Geometry check sheet. Reference: the model listing, model coordinates, mm. Round coordinates to 2 decimals unless told otherwise and drop trailing zeros. Write each loop counter-clockwise with the first axis right and the second up, starting at its lowest first coordinate (ties: lowest second). Pieces come first, ordered by that corner, then holes. Notation, with made-up numbers: M 74,89 L 96,89 A22 ccw 96,110 Z; hole C 28,37 d7. An arc over 180 degrees is marked long. Use a Markdown table: item, result.
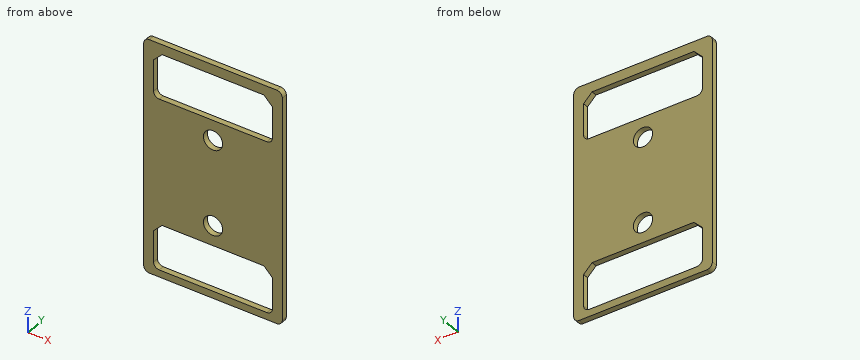
Autodesk Inventor part; units mm, degrees
ref_plane "YZ Plane" through (0, 0, 0) normal (1, 0, 0) x (0, 1, 0)
ref_plane "XZ Plane" through (0, 0, 0) normal (0, 1, 0) x (-1, 0, 0)
ref_plane "XY Plane" through (0, 0, 0) normal (0, 0, 1) x (1, 0, 0)
sketch "Sketch1" plane through (0, 0, 0) normal (0, 1, 0) x (-1, 0, 0)
  line L0 (-11.25, -20.5) -> (11.25, -20.5)
  line L1 (12.25, -19.5) -> (12.25, 19.5)
  line L2 (11.25, 20.5) -> (-11.25, 20.5)
  line L3 (-12.25, 19.5) -> (-12.25, -19.5)
  line L4 (-12.25, -20.5) -> (12.25, 20.5) construction
  line L5 (12.25, -20.5) -> (-12.25, 20.5) construction
  arc A0 (12.25, 19.5) -> (11.25, 20.5) centre (11.25, 19.5) ccw
  arc A1 (-11.25, 20.5) -> (-12.25, 19.5) centre (-11.25, 19.5) ccw
  arc A2 (-12.25, -19.5) -> (-11.25, -20.5) centre (-11.25, -19.5) ccw
  arc A3 (11.25, -20.5) -> (12.25, -19.5) centre (11.25, -19.5) ccw
  point P0 (0, 0)
  dimension "d0" = 24.5
  dimension "d1" = 41
  dimension "d2" = 1
extrude "Extrusion1" add sketch "Sketch1" along normal blind 1
sketch "Sketch2" plane through (0, 1, 0) normal (0, 1, 0) x (1, 0, 0)
  line L0 (9.5, -10.75) -> (-9.5, -10.75)
  line L1 (-10.5, -11.75) -> (-10.5, -17.25)
  line L2 (-9, -18.75) -> (9, -18.75)
  line L3 (10.5, -17.25) -> (10.5, -11.75)
  line L4 (10.5, -10.75) -> (-10.5, -18.75) construction
  line L5 (-10.5, -10.75) -> (10.5, -18.75) construction
  line L6 (-9.5, 19.25) -> (9.5, 19.25)
  line L7 (10.5, 18.25) -> (10.5, 12.75)
  line L8 (9, 11.25) -> (-9, 11.25)
  line L9 (-10.5, 12.75) -> (-10.5, 18.25)
  line L10 (-10.5, 19.25) -> (10.5, 11.25) construction
  line L11 (10.5, 19.25) -> (-10.5, 11.25) construction
  line L12 (11.25, 20.5) -> (-11.25, 20.5)
  arc A0 (-9.5, -10.75) -> (-10.5, -11.75) centre (-9.5, -11.75) ccw
  arc A1 (10.5, -11.75) -> (9.5, -10.75) centre (9.5, -11.75) ccw
  arc A2 (-9.5, 19.25) -> (-10.5, 18.25) centre (-9.5, 18.25) ccw
  arc A3 (10.5, 18.25) -> (9.5, 19.25) centre (9.5, 18.25) ccw
  line L13 (10.5, -17.25) -> (9, -18.75)
  line L14 (10.5, 12.75) -> (9, 11.25)
  line L15 (-9, -18.75) -> (-10.5, -17.25)
  line L16 (-9, 11.25) -> (-10.5, 12.75)
  point P0 (0, 0)
  point P1 (0, -14.75)
  point P2 (0, 15.25)
  dimension "d5" = 30
  dimension "d8" = 1.25
  dimension "d9" = 8
  dimension "d10" = 8
  dimension "d11" = 21
  dimension "d12" = 21
  dimension "d14" = 1.5
  dimension "d15" = 1.5
  dimension "d16" = 1.5
  dimension "d17" = 1.5
  dimension "d18" = 1.5
  dimension "d19" = 1.5
  dimension "d20" = 1.5
  dimension "d21" = 1
  dimension "d22" = 1
extrude "Extrusion2" cut sketch "Sketch2" against normal through all
sketch "Sketch3" plane through (0, 1, 0) normal (0, 1, 0) x (1, 0, 0)
  line L0 (11.25, 20.5) -> (-11.25, 20.5)
  point P0 (0, 0)
  point P1 (0, -7.24)
  point P2 (0, 7.76)
  dimension "d23" = 15
  dimension "d24" = 12.74
hole "Hole1" at (0, 1, 7.24) at (0, 1, -7.76) direction (0, -1, 0) diameter 3.4 depth 7.9 tip angle 118
equation "\"d10\" = d9"
equation "\"d12\" = d11"
equation "\"d15\" = d14"
equation "\"d16\" = d14"
equation "\"d17\" = d15"
equation "\"d18\" = d15"
equation "\"d19\" = d14"
equation "\"d20\" = d15"
properties part number "flex clamp V1" material "Stainless Steel"
Item 1: Cross-section at B-B, the plane x = 0. Record the cut outline in (y, z), and give its area (3 significant figures).
Outcome:
| item | result |
|---|---|
| outline | M 0,-20.5 L 1,-20.5 L 1,-19.25 L 0,-19.25 Z; M 0,-11.25 L 1,-11.25 L 1,-9.46 L 0,-9.46 Z; M 0,-6.06 L 1,-6.06 L 1,5.54 L 0,5.54 Z; M 0,8.94 L 1,8.94 L 1,10.75 L 0,10.75 Z; M 0,18.75 L 1,18.75 L 1,20.5 L 0,20.5 Z |
| area | 18.2 mm2 |
Item 2: Cross-section at D-D, the plane y = 0.4. Record the cut outline in (x, z).
Outcome:
| item | result |
|---|---|
| outline | M -12.25,-19.5 A1 ccw -11.25,-20.5 L 11.25,-20.5 A1 ccw 12.25,-19.5 L 12.25,19.5 A1 ccw 11.25,20.5 L -11.25,20.5 A1 ccw -12.25,19.5 Z; hole M -10.5,-18.25 A1 ccw -9.5,-19.25 L 9.5,-19.25 A1 ccw 10.5,-18.25 L 10.5,-12.75 L 9,-11.25 L -9,-11.25 L -10.5,-12.75 Z; hole M -10.5,11.75 A1 ccw -9.5,10.75 L 9.5,10.75 A1 ccw 10.5,11.75 L 10.5,17.25 L 9,18.75 L -9,18.75 L -10.5,17.25 Z; hole C 0,-7.76 d3.4; hole C 0,7.24 d3.4 |
Item 3: Go/stop test with a flat-tipped pin: pin 1 (2 mm diameter, centred on x = -7, z = 0, fed in from -Y). Record where the tip stops, or that it passes through.
Outcome:
| item | result |
|---|---|
| pin 1 | stops at y = 0 |
Item 4: Material ranges on line 1 along Z through (x, y) = (-5.5, 0.8); line 2 along Z through (x, y) = (0, 0.5); line 3 along X through (y, z) = (0.6, 7.24), recorded low to high. Write a range as from..to.
Outcome:
| item | result |
|---|---|
| line 1 | z = -20.5..-19.25, -11.25..10.75, 18.75..20.5 |
| line 2 | z = -20.5..-19.25, -11.25..-9.46, -6.06..5.54, 8.94..10.75, 18.75..20.5 |
| line 3 | x = -12.25..-1.7, 1.7..12.25 |
Item 5: Cross-section at C-C, the plane x = 4.5. Record the cut outline in (y, z), and give its area (3 significant figures).
Outcome:
| item | result |
|---|---|
| outline | M 0,-20.5 L 1,-20.5 L 1,-19.25 L 0,-19.25 Z; M 0,-11.25 L 1,-11.25 L 1,10.75 L 0,10.75 Z; M 0,18.75 L 1,18.75 L 1,20.5 L 0,20.5 Z |
| area | 25.0 mm2 |
Item 6: Cross-section at A-A, the plane z = -7.76. Record the cut outline in (x, y).
Outcome:
| item | result |
|---|---|
| outline | M -12.25,0 L -1.7,0 L -1.7,1 L -12.25,1 Z; M 1.7,0 L 12.25,0 L 12.25,1 L 1.7,1 Z |
